from build123d import *

# Parameters (mm, degrees)
SKETCH1_W                      = 38.1
SKETCH1_H                      = 1.5875
BOSS_EXTRUDE1_DEPTH            = 44.45
SKETCH2_W                      = 38.1
SKETCH2_H                      = 1.5875
BOSS_EXTRUDE2_DEPTH            = 38.1
SKETCH3_R                      = 13.208
CUT_EXTRUDE1_DEPTH             = 71.728425377
F_1_8_0_125_DIAMETER_HOLE3_D   = 3.175
F_1_8_0_125_DIAMETER_HOLE4_D   = 3.175
F_2_9_2_9_DIAMETER_HOLE1_D     = 2.9
F_2_9_2_9_DIAMETER_HOLE1_DEPTH = 3.556
F_2_9_2_9_DIAMETER_HOLE1_TIP   = 0.871247898


with BuildPart() as part:
    # Sketch1 → Boss-Extrude1 (new body)
    with BuildSketch(Plane.XY):
        with Locations((19.05, 0.79375)):
            Rectangle(SKETCH1_W, SKETCH1_H)
    extrude(amount=BOSS_EXTRUDE1_DEPTH)

    # Sketch2 → Boss-Extrude2 (add)
    with BuildSketch(Plane(origin=(0, 1.5875, 0), x_dir=(1, 0, 0), z_dir=(0, 1, 0))):
        with Locations((19.05, -0.79375)):
            Rectangle(SKETCH2_W, SKETCH2_H)
    extrude(amount=BOSS_EXTRUDE2_DEPTH)

    # Sketch3 → Cut-Extrude1 (cut, through all)
    with BuildSketch(Plane(origin=(0, 0, 0), x_dir=(-1, 0, 0), z_dir=(0, 0, -1))):
        with Locations((-19.05, 20.1295)):
            Circle(SKETCH3_R)
    extrude(amount=-CUT_EXTRUDE1_DEPTH, mode=Mode.SUBTRACT)

    # 1/8 (0.125) Diameter Hole3 (through all)
    with Locations(Plane(origin=(0, 0, 0), x_dir=(-1, 0, 0), z_dir=(0, 0, -1))):
        with Locations((-35.56, 20.1295), (-10.795, 34.427579416), (-2.54, 20.1295), (-10.795, 5.831420584)):
            Hole(F_1_8_0_125_DIAMETER_HOLE3_D / 2)

    # 1/8 (0.125) Diameter Hole4 (through all)
    with Locations(Plane(origin=(0, 1.5875, 0), x_dir=(1, 0, 0), z_dir=(0, 1, 0))):
        with Locations((34.29, -12.7), (21.59, -12.7), (21.59, -35.56), (34.29, -35.469930371)):
            Hole(F_1_8_0_125_DIAMETER_HOLE4_D / 2)

    # Ø2.9 (2.9) Diameter Hole1
    with Locations(Plane(origin=(0, 0, 0), x_dir=(-1, 0, 0), z_dir=(0, 0, -1))):
        with Locations((-27.305, 5.831420584), (-27.305, 34.427579416)):
            Hole(F_2_9_2_9_DIAMETER_HOLE1_D / 2, depth=F_2_9_2_9_DIAMETER_HOLE1_DEPTH)
            with Locations((0, 0, -(F_2_9_2_9_DIAMETER_HOLE1_DEPTH + F_2_9_2_9_DIAMETER_HOLE1_TIP / 2))):  # 118° drill point
                Cone(0, F_2_9_2_9_DIAMETER_HOLE1_D / 2, F_2_9_2_9_DIAMETER_HOLE1_TIP, mode=Mode.SUBTRACT)


solid = part.part
Verification items for the finished model (mm, model axes). A direction names the side the tool comes from. Give positions to 0.01 mm unless a question says otherwise; leave off trailing zeros. Write each loop counter-clockwise with the first axis right and the second up, starting at its lowest first coordinate (ties: lowest second). Pieces come first, ordered by that corner, then holes. Notation, with made-up numbers: (-28, 84.5) - (-7, 84.5) arc R20 cw to (-7, 110.5) - close; hole circle Ø4 at (28, -38). An arc over 180 degrees is marked (long way). Answer as CSV lines item,"result". Start each with the question number.
1. Thickness scan on line 1 (X direction, y = 0.4, z = 12.7); line 2 (Z direction, x = 21.59, y = 0.8); line 3 (X direction, y = 1, z = 35). Record the ranges inside material, lowest first.
2. Sectioned sample at C-C (y = 5). Record the boundary of the cut face in (x, z), then the cut area to 3 significant figures.
3. Sectioned sample at A-A (z = 12.7). Record the boundary of the cut face in (x, y).
4. Draft check along Y on faces 1 (the face through (6, 24, 0)), 2 (the face through (12.31, 6.31, 0.8)), 3 (the face through (19, 0, 22)). Enter one of: pulls with the +Y half, pulls with the -Y half, needs draft (parallel to the pull), parting line crosses it, or undercut.
5. Sectioned sample at B-B (x = 19.05). Record the boundary of the cut face in (y, z).
6. Depth check by flat-ended pin: pin 1 (6 mm diameter, centred on x = 24, y = 4.5, fed in from -Z); pin 2 (1.9 mm diameter, centred on x = 21.59, z = 35.56, fed in from +Y); pin 3 (8 mm diameter, centred on x = 8.5, z = 27.5, fed in from +Y). Enter the tip coordinate at first touch or a pass-through.
7. Sectioned sample at D-D (y = 29.5). Record the boundary of the cut face in (x, z), then the cut area to 3 significant figures.
8. Set-up check for faces 4 (the face through (11.53, 33.02, 0.8)), 5 (the face through (19, 1.588, 23)): record each of +Z, -Z, +X, -X, +Y, -Y from which the full face is reachable in a straight line by a thin tool's end or side.
Derived:
1,line 1,"0 to 20, 23.18 to 32.7, 35.88 to 38.1"
1,line 2,"0 to 11.11, 14.29 to 33.97, 37.15 to 44.45"
1,line 3,"0 to 20.1, 23.08 to 32.77, 35.81 to 38.1"
2,outline,"(0, 0) - (9.44, 0) - (9.44, 1.59) - (0, 1.59) - close; (12.15, 0) - (26.12, 0) - (26.12, 1.59) - (12.15, 1.59) - close; (28.49, 0) - (38.1, 0) - (38.1, 1.59) - (28.49, 1.59) - close"
2,area,"52.4 mm²"
3,outline,"(0, 0) - (20, 0) - (20, 1.59) - (0, 1.59) - close; (23.18, 0) - (32.7, 0) - (32.7, 1.59) - (23.18, 1.59) - close; (35.88, 0) - (38.1, 0) - (38.1, 1.59) - (35.88, 1.59) - close"
4,face 1,"needs draft"
4,face 2,"undercut"
4,face 3,"pulls with the -Y half"
5,outline,"(0, 0) - (6.92, 0) - (6.92, 1.59) - (1.59, 1.59) - (1.59, 44.45) - (0, 44.45) - close; (33.34, 0) - (39.69, 0) - (39.69, 1.59) - (33.34, 1.59) - close"
6,pin 1,"z = 0"
6,pin 2,"through"
6,pin 3,"y = 1.59"
7,outline,"(0, 0) - (9.74, 0) - (9.74, 1.59) - (0, 1.59) - close; (28.36, 0) - (38.1, 0) - (38.1, 1.59) - (28.36, 1.59) - close"
7,area,"30.9 mm²"
8,face 4,"+Z, -Z"
8,face 5,"+Z, +X, -X, +Y"
